Geometry check sheet. Reference: the model listing, model coordinates, mm. Face numbers are marked on the shaded views. Coordinates: 2 decimals unless noted, no trailing zeros. Write each loop counter-clockwise with the first axis right and the second up, starting at its lowest first coordinate (ties: lowest second). Pieces come first, ordered by that corner, then holes.
from build123d import *

# Parameters (mm, degrees)
CROQUIS1_W            = 5.35
CROQUIS1_H            = 7.8
CROQUIS4_R            = 3.5
CORTAR_EXTRUIR1_DEPTH = 8
CROQUIS3_W            = 1.2
CROQUIS3_H            = 6.6
REDONDEO1_R           = 0.2
REDONDEO2_R           = 0.2
REDONDEO3_R           = 0.2


with BuildPart() as part:
    # Croquis1 → Revolución1 (revolve)
    with BuildSketch(Plane(origin=(0, 0, 0), x_dir=(1, 0, 0), z_dir=(0, 1, 0))):
        with Locations((2.675, 3.9)):
            Rectangle(CROQUIS1_W, CROQUIS1_H)
    revolve(axis=Axis((0, 0, 0), (0, 0, -1)))

    # Croquis4 → Cortar-Extruir1 (cut)
    with BuildSketch(Plane(origin=(0, 0, -7.8), x_dir=(-1, 0, 0), z_dir=(0, 0, -1))):
        Circle(CROQUIS4_R)
    extrude(amount=-CORTAR_EXTRUIR1_DEPTH, mode=Mode.SUBTRACT)

    # Croquis3 → Cortar-Revolución1 (revolve, cut)
    with BuildSketch(Plane(origin=(0, 0, 0), x_dir=(1, 0, 0), z_dir=(0, 1, 0))):
        with Locations((4.75, 4.5)):
            Rectangle(CROQUIS3_W, CROQUIS3_H)
    revolve(axis=Axis((0, 0, -1.2), (0, 0, -1)), mode=Mode.SUBTRACT)

    # Redondeo1
    redondeo1_edges = [part.edges().sort_by_distance(p)[0] for p in [
        (-4.15, 0, -7.8),
    ]]
    fillet(redondeo1_edges, radius=REDONDEO1_R)

    # Redondeo2
    redondeo2_edges = [part.edges().sort_by_distance(p)[0] for p in [
        (-4.15, 0, -1.2),
    ]]
    fillet(redondeo2_edges, radius=REDONDEO2_R)

    # Redondeo3
    redondeo3_edges = [part.edges().sort_by_distance(p)[0] for p in [
        (-5.35, 0, -1.2),
        (-5.35, 0, 0),
    ]]
    fillet(redondeo3_edges, radius=REDONDEO3_R)


solid = part.part
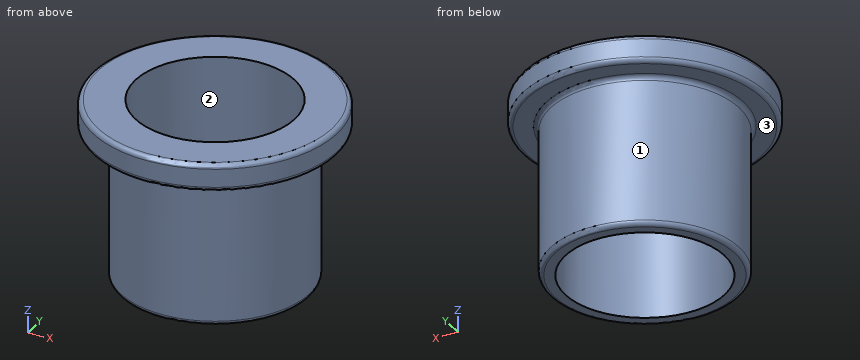
1. Thickness scan on line 1 along Y through (x, z) = (0, -5); line 2 along Z through (x, y) = (3, 3.5); line 3 along X through (y, z) = (-3, -7). Record the ranges inside material, lowest first.
Computed values:
line 1: y = -4.15 to -3.5, 3.5 to 4.15
line 2: z = -1.2 to 0
line 3: x = -2.87 to -1.8, 1.8 to 2.87
2. Draft check along Y on the marked faces 1, 2 and 3. Enter one of: released by +Y, released by -Y, zero draft, split by the parting line, or undercut.
Computed values:
face 1: split by the parting line
face 2: undercut
face 3: zero draft
3. Sectioned sample at C-C, the plane z = -4. Record the boundary of the cut face in (x, y).
Computed values:
outline: circle Ø8.3 at (0, 0); hole circle Ø7 at (0, 0)
4. Sectioned sample at A-A, the plane y = 0. Record the boundary of the cut face in (x, z).
Computed values:
outline: (-5.35, -1) arc R0.2 ccw to (-5.15, -1.2) - (-4.35, -1.2) arc R0.2 cw to (-4.15, -1.4) - (-4.15, -7.6) arc R0.2 ccw to (-3.95, -7.8) - (-3.5, -7.8) - (-3.5, 0) - (-5.15, 0) arc R0.2 ccw to (-5.35, -0.2) - close; (3.5, -7.8) - (3.95, -7.8) arc R0.2 ccw to (4.15, -7.6) - (4.15, -1.4) arc R0.2 cw to (4.35, -1.2) - (5.15, -1.2) arc R0.2 ccw to (5.35, -1) - (5.35, -0.2) arc R0.2 ccw to (5.15, 0) - (3.5, 0) - close
5. Gauge pin test, flat ends, axial feed: pin 1 Ø4 at (x, z) = (1.5, -6) entering from +Y; pin 2 Ø1.5 at (y, z) = (-3.5, -4) entering from -X; pin 3 Ø1 at (y, z) = (-1, -3) entering from -X. Record the tip position at first contact, or that the pin passes through.
Computed values:
pin 1: stops at y = 4.15
pin 2: stops at x = -3.11
pin 3: stops at x = -4.12
